The listing builds one solid part. Answer for the finished solid, in the listing's coordinates (mm). Face numbers are marked on the shaded views. A direction names the side the tool comes from. Coordinates: 2 decimals unless noted, no trailing zeros. Order: outer loops, then holes, each group sorted by start corner. A loop starts at its lowest first (then second) coordinate and runs counter-clockwise, first axis right, second up. Notation, with made-up numbers: (52, -35.75) -> (105, -35.75) arc R30 cw to (105, 0.25) -> close; hole circle Ø9 at (46, 20). An arc over 180 degrees is marked (long way). Return JSON: item names as keys, results as strings.
from build123d import *

# Parameters (mm, degrees)
F2_R          = 1.25
F3_DEPTH      = 29.001
F3_DEPTH_BACK = 25


with BuildPart() as f1:
    # F0 (on Front) → F1 (revolve)
    with BuildSketch(Plane.XZ):
        Polygon((21, 21.2053321302), (21, 10), (29, 10), (29, 12.4697282932), (23.756984706, 21.2053321302), align=None)
        Polygon((21, 25.7988579593), (21, 21.2053321302), (23.756984706, 21.2053321302), align=None)
        Polygon((15.5, 30), (15.5, 0), (21, 0), (21, 10), (21, 21.2053321302), (21, 25.7988579593), (21, 30), align=None)
    revolve(axis=Axis((0, 0, 17.8434439003), (0, 0, 1)))

    # F2 (on Right) → F3 (cut, two sides)
    with BuildSketch(Plane.YZ) as f3_sk:
        with Locations((0, 27.5)):
            Circle(F2_R)
    extrude(amount=-F3_DEPTH, mode=Mode.SUBTRACT)
    extrude(f3_sk.sketch, amount=F3_DEPTH_BACK, mode=Mode.SUBTRACT)


solid = f1.part
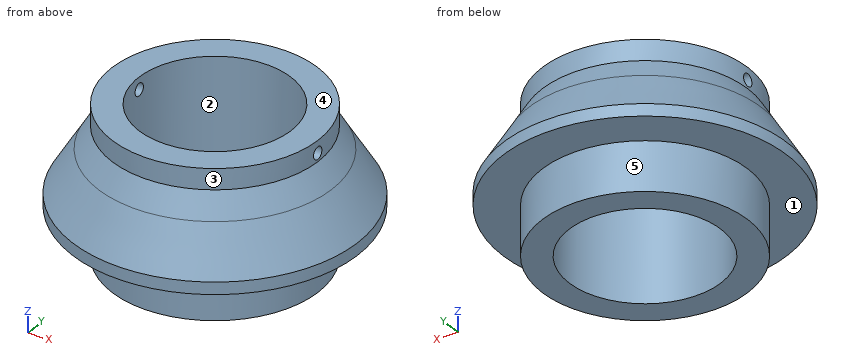
1. Each of these flat-tipped pins is pushed along its axis until it touches: pin 1 Ø6 at (y, z) = (-20.5, 8) entering from +X; pin 2 Ø5 at (y, z) = (13.5, 26) entering from -X; pin 3 Ø1.5 at (y, z) = (-20.5, 12) entering from +X. Where does it stop, or does it pass through?
Answer block:
{"pin 1": "stops at x = 22.53", "pin 2": "stops at x = -18.54", "pin 3": "stops at x = 21.24"}
2. For the marked faces 4 and 5, determine the directions among +Z, -Z, +X, -X, +Y, -Y from which every point of the face is accessible in a straight line to the end or side of a thin tool.
Answer block:
{"face 4": "+Z, +X, -X, +Y, -Y", "face 5": "-Z"}
3. The part is cut by section C-C on z = 11.5. Give the vertices of the cut face in (x, y).
Answer block:
{"outline": "circle Ø58 at (0, 0); hole circle Ø31 at (0, 0)"}
4. The part is cut by section A-A on z = 27.5. Give the vertices of the cut face in (x, y), and give its area (3 significant figures).
Answer block:
{"outline": "(-20.96, -1.25) arc R21 ccw to (20.96, -1.25) -> (15.45, -1.25) arc R15.5 cw to (-15.45, -1.25) -> close; (-20.96, 1.25) -> (-15.45, 1.25) arc R15.5 cw to (15.45, 1.25) -> (20.96, 1.25) arc R21 ccw to start", "area": "603 mm2"}
5. Consider line 1 (Z direction, x = 18.15, y = 0); line 2 (X direction, y = -10.5, z = 19.5); line 3 (Y direction, x = 2, z = 8.5). Determine where each line is inside the solid, lowest interval first. Write a range as from..to.
Answer block:
{"line 1": "z = 0..26.25, 28.75..30", "line 2": "x = -22.45..-11.4, 11.4..22.45", "line 3": "y = -20.9..-15.37, 15.37..20.9"}
6. Determine the mould class of the marked faces 1, 2 and 3 for opening direction Y: pulls with the +Y half, pulls with the -Y half, needs draft (parallel to the pull), parting line crosses it, or undercut.
Answer block:
{"face 1": "needs draft", "face 2": "undercut", "face 3": "parting line crosses it"}
7. The part is cut by section B-B on z = 7. Give the vertices of the cut face in (x, y), and give its area (3 significant figures).
Answer block:
{"outline": "circle Ø42 at (0, 0); hole circle Ø31 at (0, 0)", "area": "631 mm2"}
